The model under review builds one solid part; all positions refer to its coordinate system, in mm. Face numbers are marked on the shaded views. A direction names the side the tool comes from. Coordinates: 2 decimals unless noted, no trailing zeros. Write each loop counter-clockwise with the first axis right and the second up, starting at its lowest first coordinate (ties: lowest second). Pieces come first, ordered by that corner, then holes.
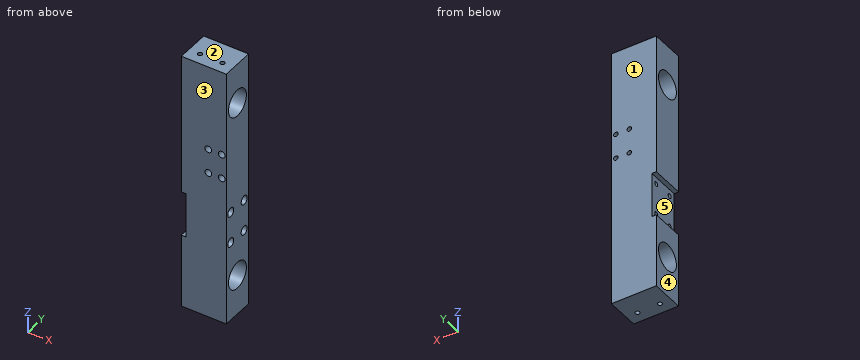
```python
from build123d import *

# Parameters (mm, degrees)
SKETCH1_W           = 20
SKETCH1_H           = 15
BOSS_EXTRUDE1_DEPTH = 116
SKETCH1_5_R         = 1
CUT_EXTRUDE1_DEPTH  = 10
SKETCH4_R           = 1
CUT_EXTRUDE2_DEPTH  = 10
SKETCH5_R           = 2.5
CUT_EXTRUDE3_DEPTH  = 21
SKETCH6_R           = 6
CUT_EXTRUDE4_DEPTH  = 21
SKETCH8_R           = 1
CUT_EXTRUDE5_DEPTH  = 16
SKETCH9_R           = 1.5
CUT_EXTRUDE6_DEPTH  = 5
SKETCH10_R          = 1
CUT_EXTRUDE7_DEPTH  = 21
SKETCH11_R          = 2
CUT_EXTRUDE8_DEPTH  = 5
SKETCH10_3_W        = 10
SKETCH10_3_H        = 7.5
SKETCH10_3_R        = 1
CUT_EXTRUDE9_DEPTH  = 2


with BuildPart() as part:
    # Sketch1 → Boss-Extrude1 (new body)
    with BuildSketch(Plane.XY):
        with Locations((10, 7.5)):
            Rectangle(SKETCH1_W, SKETCH1_H)
    extrude(amount=BOSS_EXTRUDE1_DEPTH)

    # Sketch1_5 → Cut-Extrude1 (cut)
    with BuildSketch(Plane.XY):
        with Locations((15, 5)):
            Circle(SKETCH1_5_R)
        with Locations((5, 5)):
            Circle(SKETCH1_5_R)
    extrude(amount=CUT_EXTRUDE1_DEPTH, mode=Mode.SUBTRACT)

    # Sketch4 → Cut-Extrude2 (cut)
    with BuildSketch(Plane.XY.offset(116)):
        with Locations((5, 5)):
            Circle(SKETCH4_R)
        with Locations((15, 5)):
            Circle(SKETCH4_R)
    extrude(amount=-CUT_EXTRUDE2_DEPTH, mode=Mode.SUBTRACT)

    # Sketch5 → Cut-Extrude3 (cut, through all)
    with BuildSketch(Plane(origin=(20, 0, 0), x_dir=(0, 0, -1), z_dir=(1, 0, 0))):
        with Locations((-98, 7.5)):
            Circle(SKETCH5_R)
        with Locations((-18, 7.5)):
            Circle(SKETCH5_R)
    extrude(amount=-CUT_EXTRUDE3_DEPTH, mode=Mode.SUBTRACT)

    # Sketch6 → Cut-Extrude4 (cut, through all)
    with BuildSketch(Plane(origin=(20, 0, 0), x_dir=(0, 0, -1), z_dir=(1, 0, 0))):
        with Locations((-98, 7.5)):
            Circle(SKETCH6_R)
        with Locations((-18, 7.5)):
            Circle(SKETCH6_R)
    extrude(amount=-CUT_EXTRUDE4_DEPTH, mode=Mode.SUBTRACT)

    # Sketch8 → Cut-Extrude5 (cut, through all)
    with BuildSketch(Plane(origin=(0, 15, 0), x_dir=(1, 0, 0), z_dir=(0, 1, 0))):
        with Locations((12, -66.8)):
            Circle(SKETCH8_R)
        with Locations((18, -66.8)):
            Circle(SKETCH8_R)
        with Locations((18, -77.8)):
            Circle(SKETCH8_R)
        with Locations((12, -77.8)):
            Circle(SKETCH8_R)
    extrude(amount=-CUT_EXTRUDE5_DEPTH, mode=Mode.SUBTRACT)

    # Sketch9 → Cut-Extrude6 (cut)
    with BuildSketch(Plane(origin=(0, 0, 0), x_dir=(-1, 0, 0), z_dir=(0, -1, 0))):
        with Locations((-18, -66.8)):
            Circle(SKETCH9_R)
        with Locations((-18, -77.8)):
            Circle(SKETCH9_R)
        with Locations((-12, -77.8)):
            Circle(SKETCH9_R)
        with Locations((-12, -66.8)):
            Circle(SKETCH9_R)
    extrude(amount=-CUT_EXTRUDE6_DEPTH, mode=Mode.SUBTRACT)

    # Sketch10 → Cut-Extrude7 (cut, through all)
    with BuildSketch(Plane.ZY):
        with Locations((36, 12)):
            Circle(SKETCH10_R)
        with Locations((50, 12)):
            Circle(SKETCH10_R)
        with Locations((50, 3)):
            Circle(SKETCH10_R)
        with Locations((36, 3)):
            Circle(SKETCH10_R)
    extrude(amount=-CUT_EXTRUDE7_DEPTH, mode=Mode.SUBTRACT)

    # Sketch11 → Cut-Extrude8 (cut)
    with BuildSketch(Plane(origin=(20, 0, 0), x_dir=(0, 0, -1), z_dir=(1, 0, 0))):
        with Locations((-36, 12)):
            Circle(SKETCH11_R)
        with Locations((-36, 3)):
            Circle(SKETCH11_R)
        with Locations((-50, 3)):
            Circle(SKETCH11_R)
        with Locations((-50, 12)):
            Circle(SKETCH11_R)
    extrude(amount=-CUT_EXTRUDE8_DEPTH, mode=Mode.SUBTRACT)

    # Sketch10_3 → Cut-Extrude9 (cut)
    with BuildSketch(Plane.ZY):
        with Locations((38, 11.25)):
            Rectangle(SKETCH10_3_W, SKETCH10_3_H)
        with Locations((36, 12)):
            Circle(SKETCH10_3_R, mode=Mode.SUBTRACT)
        with Locations((48, 11.25)):
            Rectangle(SKETCH10_3_W, SKETCH10_3_H)
        with Locations((50, 12)):
            Circle(SKETCH10_3_R, mode=Mode.SUBTRACT)
        with Locations((48, 3.75)):
            Rectangle(SKETCH10_3_W, SKETCH10_3_H)
        with Locations((50, 3)):
            Circle(SKETCH10_3_R, mode=Mode.SUBTRACT)
        with Locations((38, 3.75)):
            Rectangle(SKETCH10_3_W, SKETCH10_3_H)
        with Locations((36, 3)):
            Circle(SKETCH10_3_R, mode=Mode.SUBTRACT)
    extrude(amount=-CUT_EXTRUDE9_DEPTH, mode=Mode.SUBTRACT)


solid = part.part
```
Item 1: Take a section at C-C, the plane z = 66.8. Write out the cut boundary in (x, y).
Solved:
outline: (0, 0) - (10.5, 0) - (10.5, 5) - (11, 5) - (11, 15) - (0, 15) - close; (13, 5) - (13.5, 5) - (13.5, 0) - (16.5, 0) - (16.5, 5) - (17, 5) - (17, 15) - (13, 15) - close; (19, 5) - (19.5, 5) - (19.5, 0) - (20, 0) - (20, 15) - (19, 15) - close
Item 2: Machinability: for the marked faces 4 and 5, which of the approach directions +Z, -Z, +X, -X, +Y, -Y give a long, thin tool a straight path to every point of the face, cutting with its end or side? Answer none if there is none.
Solved:
face 4: +Z, -Z, -X, +Y, -Y
face 5: -X, +Y, -Y
Item 3: Take a section at B-B, the plane z = 18. Write out the cut boundary in (x, y), plus the area to 3 significant figures.
Solved:
outline: (0, 0) - (20, 0) - (20, 1.5) - (0, 1.5) - close; (0, 13.5) - (20, 13.5) - (20, 15) - (0, 15) - close
area: 60.0 mm2
Item 4: To check wall thickness, follow line 1 along X through (y, z) = (2.05, 77.8); line 2 along X through (y, z) = (11.5, 77.8); line 3 along Z through (x, y) = (10.5, 7.25). State the ranges of each line that lie inside material, in increasing order.
Solved:
line 1: x = 0 to 10.5, 13.5 to 16.5, 19.5 to 20
line 2: x = 0 to 11, 13 to 17, 19 to 20
line 3: z = 0 to 12.01, 23.99 to 92.01, 103.99 to 116
Item 5: Mouldability with a two-part tool opening along Y and no side actions: class the marked faces 1, 2 and 3 as pulls with the +Y half, pulls with the -Y half, needs draft (parallel to the pull), parting line crosses it, or undercut.
Solved:
face 1: pulls with the +Y half
face 2: needs draft
face 3: pulls with the -Y half
Item 6: For pin 1 (2.5 mm diameter, centred on y = 12, z = 36, fed in from +X); pin 2 (3.5 mm diameter, centred on x = 18, z = 66.8, fed in from -Y); pin 3 (0.6 mm diameter, centred on x = 15.5, y = 5, fed in from +Z); pin 4 (0.6 mm diameter, centred on x = 15, y = 5.5, fed in from -Z), all flat-tipped, find the tip position at first contact; note any pin that passes through.
Solved:
pin 1: stops at x = 15
pin 2: stops at y = 0
pin 3: stops at z = 106
pin 4: stops at z = 10
Item 7: Take a section at A-A, the plane x = 12. Count the separate pieces of the cut face and the enclosed holes in it, plus the area to 3 significant figures.
Solved:
separate pieces: 3
enclosed holes: 6
area: 1,430 mm2
